Geometry: final body of the model. Coordinates: model frame, mm. A direction names the side the tool comes from. Give positions to 0.01 mm unless a question says otherwise; leave off trailing zeros. Write each loop counter-clockwise with the first axis right and the second up, starting at its lowest first coordinate (ties: lowest second). Pieces come first, ordered by that corner, then holes. Notation, with made-up numbers: (67.5, -30) - (101.5, -30) arc R7 cw to (101.5, -23) - close; hole circle Ø10 at (31.25, 76). An arc over 180 degrees is marked (long way). Return JSON: item names as keys, results as strings.
from build123d import *

# Parameters (mm, degrees)
CYLINDER_R     = 6.5
CYLINDER_DEPTH = 0.3
BOX001_W       = 1
BOX001_H       = 2
BOX001_DEPTH   = 1
BOX002_W       = 3
BOX002_H       = 4
BOX002_DEPTH   = 1
BOX003_W       = 1
BOX003_H       = 2
BOX003_DEPTH   = 1
BOX004_W       = 1
BOX004_H       = 1
BOX004_DEPTH   = 1
BOX005_W       = 1
BOX005_H       = 5
BOX005_DEPTH   = 1
BOX006_W       = 1
BOX006_H       = 5
BOX006_DEPTH   = 1
BOX007_W       = 1
BOX007_H       = 2
BOX007_DEPTH   = 1
BOX008_W       = 1
BOX008_H       = 2
BOX008_DEPTH   = 1
BOX009_W       = 1
BOX009_H       = 2
BOX009_DEPTH   = 1
BOX010_W       = 1
BOX010_H       = 2
BOX010_DEPTH   = 1
BOX011_W       = 1
BOX011_H       = 3
BOX011_DEPTH   = 1
BOX012_W       = 1
BOX012_H       = 3
BOX012_DEPTH   = 1
BOX013_W       = 1
BOX013_H       = 2
BOX013_DEPTH   = 1
BOX014_W       = 1
BOX014_H       = 2
BOX014_DEPTH   = 1
BOX_W          = 1
BOX_H          = 1
BOX_DEPTH      = 1


with BuildPart() as cilindro:
    # Cylinder → Cylinder (new body)
    with BuildSketch(Plane(origin=(3.5, -4, 0), x_dir=(1, 0, 0), z_dir=(0, 0, 1))):
        Circle(CYLINDER_R)
    extrude(amount=CYLINDER_DEPTH)


with BuildPart() as cubo001:
    # Box001 → Box001 (new body)
    with BuildSketch(Plane(origin=(1, -2, 0), x_dir=(1, 0, 0), z_dir=(0, 0, 1))):
        with Locations((0.5, 1)):
            Rectangle(BOX001_W, BOX001_H)
    extrude(amount=BOX001_DEPTH)


with BuildPart() as cubo002:
    # Box002 → Box002 (new body)
    with BuildSketch(Plane(origin=(2, -5, 0), x_dir=(1, 0, 0), z_dir=(0, 0, 1))):
        with Locations((1.5, 2)):
            Rectangle(BOX002_W, BOX002_H)
    extrude(amount=BOX002_DEPTH)


with BuildPart() as cubo003:
    # Box003 → Box003 (new body)
    with BuildSketch(Plane(origin=(5, -2, 0), x_dir=(1, 0, 0), z_dir=(0, 0, 1))):
        with Locations((0.5, 1)):
            Rectangle(BOX003_W, BOX003_H)
    extrude(amount=BOX003_DEPTH)


with BuildPart() as cubo004:
    # Box004 → Box004 (new body)
    with BuildSketch(Plane(origin=(6, 0, 0), x_dir=(1, 0, 0), z_dir=(0, 0, 1))):
        with Locations((0.5, 0.5)):
            Rectangle(BOX004_W, BOX004_H)
    extrude(amount=BOX004_DEPTH)


with BuildPart() as cubo005:
    # Box005 → Box005 (new body)
    with BuildSketch(Plane(origin=(0, -6, 0), x_dir=(1, 0, 0), z_dir=(0, 0, 1))):
        with Locations((0.5, 2.5)):
            Rectangle(BOX005_W, BOX005_H)
    extrude(amount=BOX005_DEPTH)


with BuildPart() as cubo006:
    # Box006 → Box006 (new body)
    with BuildSketch(Plane(origin=(6, -6, 0), x_dir=(1, 0, 0), z_dir=(0, 0, 1))):
        with Locations((0.5, 2.5)):
            Rectangle(BOX006_W, BOX006_H)
    extrude(amount=BOX006_DEPTH)


with BuildPart() as cubo007:
    # Box007 → Box007 (new body)
    with BuildSketch(Plane(origin=(1, -5, 0), x_dir=(1, 0, 0), z_dir=(0, 0, 1))):
        with Locations((0.5, 1)):
            Rectangle(BOX007_W, BOX007_H)
    extrude(amount=BOX007_DEPTH)


with BuildPart() as cubo008:
    # Box008 → Box008 (new body)
    with BuildSketch(Plane(origin=(5, -5, 0), x_dir=(1, 0, 0), z_dir=(0, 0, 1))):
        with Locations((0.5, 1)):
            Rectangle(BOX008_W, BOX008_H)
    extrude(amount=BOX008_DEPTH)


with BuildPart() as cubo009:
    # Box009 → Box009 (new body)
    with BuildSketch(Plane(origin=(-1, -4, 0), x_dir=(1, 0, 0), z_dir=(0, 0, 1))):
        with Locations((0.5, 1)):
            Rectangle(BOX009_W, BOX009_H)
    extrude(amount=BOX009_DEPTH)


with BuildPart() as cubo010:
    # Box010 → Box010 (new body)
    with BuildSketch(Plane(origin=(7, -4, 0), x_dir=(1, 0, 0), z_dir=(0, 0, 1))):
        with Locations((0.5, 1)):
            Rectangle(BOX010_W, BOX010_H)
    extrude(amount=BOX010_DEPTH)


with BuildPart() as cubo011:
    # Box011 → Box011 (new body)
    with BuildSketch(Plane(origin=(-2, -6, 0), x_dir=(1, 0, 0), z_dir=(0, 0, 1))):
        with Locations((0.5, 1.5)):
            Rectangle(BOX011_W, BOX011_H)
    extrude(amount=BOX011_DEPTH)


with BuildPart() as cubo012:
    # Box012 → Box012 (new body)
    with BuildSketch(Plane(origin=(8, -6, 0), x_dir=(1, 0, 0), z_dir=(0, 0, 1))):
        with Locations((0.5, 1.5)):
            Rectangle(BOX012_W, BOX012_H)
    extrude(amount=BOX012_DEPTH)


with BuildPart() as cubo013:
    # Box013 → Box013 (new body)
    with BuildSketch(Plane(origin=(3, -7, 0), x_dir=(0, 1, 0), z_dir=(0, 0, 1))):
        with Locations((0.5, 1)):
            Rectangle(BOX013_W, BOX013_H)
    extrude(amount=BOX013_DEPTH)


with BuildPart() as cubo014:
    # Box014 → Box014 (new body)
    with BuildSketch(Plane(origin=(6, -7, 0), x_dir=(0, 1, 0), z_dir=(0, 0, 1))):
        with Locations((0.5, 1)):
            Rectangle(BOX014_W, BOX014_H)
    extrude(amount=BOX014_DEPTH)


with BuildPart() as fusion001:
    # Box → Box (new body)
    with BuildSketch(Plane.XY):
        with Locations((0.5, 0.5)):
            Rectangle(BOX_W, BOX_H)
    extrude(amount=BOX_DEPTH)

    # Fusion: union Cubo001, Cubo002, Cubo003, Cubo004, Cubo005, Cubo006, Cubo007, Cubo008, Cubo009, Cubo010, Cubo011, Cubo012, Cubo013, Cubo014
    add(cubo001.part)
    add(cubo002.part)
    add(cubo003.part)
    add(cubo004.part)
    add(cubo005.part)
    add(cubo006.part)
    add(cubo007.part)
    add(cubo008.part)
    add(cubo009.part)
    add(cubo010.part)
    add(cubo011.part)
    add(cubo012.part)
    add(cubo013.part)
    add(cubo014.part)

    # Fusion001: union Cilindro
    add(cilindro.part)


solid = fusion001.part
Q1. Pin query (flat end, axial travel): P1, Ø0.6, axis at y = -4.5, z = 1, coming from the +X side; P2, Ø0.6, axis at y = -5.5, z = 0.5, coming from the +X side; P3, Ø0.6, axis at x = 0.5, z = 0.5, coming from the +Y side. Return the tip coordinate at first contact, or that it passes through.
Answer key:
{"P1": "stops at x = 9", "P2": "stops at x = 9.87", "P3": "stops at y = 1.88"}
Q2. Mould query, pull axis X, two halves, no side actions, for faces 3 (the flat face through (6.5, 0.5, 1)), 4 (the flat face through (1.5, -2.5, 0.3)). Classes: pulls with the +X half, pulls with the -X half, needs draft (parallel to the pull), parting line crosses it, or undercut.
Answer key:
{"face 3": "needs draft", "face 4": "undercut"}
Q3. Set-up query: faces 1 (the flat face through (5.5, -2.5, 0.3)), 2 (the flat face through (3, -4, 1)). Return all of +Z, -Z, +X, -X, +Y, -Y with unobstructed straight access to the full face (end or side cutting, diameter ignored); none if empty.
Answer key:
{"face 1": "+Z", "face 2": "+Z, +X, -X, +Y, -Y"}
Q4. Section query D-D, the plane x = 0.5. Return the cut outline in (y, z).
Answer key:
{"outline": "(-9.77, 0) - (1.77, 0) - (1.77, 0.3) - (1, 0.3) - (1, 1) - (0, 1) - (0, 0.3) - (-1, 0.3) - (-1, 1) - (-6, 1) - (-6, 0.3) - (-9.77, 0.3) - close"}
Q5. Material intervals for probe 1 along Y at (x, z) = (1.75, 0.85); probe 2 along X at (y, z) = (-2.75, 0.65); probe 3 along X at (y, z) = (-5.75, 0.35), sorted ascending. Write a range as [from, to].
Answer key:
{"probe 1": "y = [-7, -6], [-5, -3], [-2, 0]", "probe 2": "x = [-1, 1], [2, 5], [6, 8]", "probe 3": "x = [-2, -1], [0, 1], [6, 7], [8, 9]"}
Q6. Section query B-B, the plane x = 3.5. Return the cut outline in (y, z), plus the area to 3 significant figures.
Answer key:
{"outline": "(-10.5, 0) - (2.5, 0) - (2.5, 0.3) - (-1, 0.3) - (-1, 1) - (-5, 1) - (-5, 0.3) - (-10.5, 0.3) - close", "area": "6.70 mm^2"}
Q7. Section query C-C, the plane y = -3.25. Return the cut outline in (x, z).
Answer key:
{"outline": "(-2.96, 0) - (9.96, 0) - (9.96, 0.3) - (9, 0.3) - (9, 1) - (-2, 1) - (-2, 0.3) - (-2.96, 0.3) - close"}
